```python
from build123d import *

# Parameters (mm, degrees)
F0_R      = 1.5
F0_R_2    = 11.7126871306
F1_DEPTH  = 4
F2_R      = 4
F3_DEPTH  = 15
F6_DEPTH  = 0.6
F7_W      = 42.3
F7_H      = 22
F8_DEPTH  = 5
F11_R     = 1.0444740365
F12_DEPTH = 5
F14_R     = 1.0444740365
F15_DEPTH = 5
F16_W     = 6.0576063115
F16_H     = 10.3428596631
F16_R     = 1.0444740365
F17_DEPTH = 6
F18_SIZE  = 5.99999
F19_R     = 1.4573614865
F20_DEPTH = 7
F21_W     = 1.9849594682
F21_H     = 5.3345812485
F22_DEPTH = 5
F23_W     = 6.0576063115
F23_H     = 5.2529345267
F24_DEPTH = 1


# Not quite as in the source:
# - a fillet or chamfer is up to 0.001 mm smaller than in the source, because OpenCascade refuses the exact size


with BuildPart() as f1:
    # F0 (on Top) → F1 (new body)
    with BuildSketch(Plane.XY):
        with BuildLine():
            Line((21.15, -21.15), (21.15, 21.15))
            Line((21.15, 21.15), (8.5471369535, 21.15))
            ThreePointArc((8.5471369535, 21.15), (6.0437384995, 27.1937384995), (0, 29.6971369535))
            ThreePointArc((0, 29.6971369535), (-6.0437384995, 27.1937384995), (-8.5471369535, 21.15))
            Line((-8.5471369535, 21.15), (-21.15, 21.15))
            Line((-21.15, 21.15), (-21.15, -21.15))
            Line((-21.15, -21.15), (-8.5471369535, -21.15))
            ThreePointArc((-8.5471369535, -21.15), (0, -29.6971369535), (8.5471369535, -21.15))
            Line((8.5471369535, -21.15), (21.15, -21.15))
        make_face()
        with Locations((-15.5, -15.5)):
            Circle(F0_R, mode=Mode.SUBTRACT)
        with Locations((15.5, -15.5)):
            Circle(F0_R, mode=Mode.SUBTRACT)
        with Locations((-15.5, 15.5)):
            Circle(F0_R, mode=Mode.SUBTRACT)
        Circle(F0_R_2, mode=Mode.SUBTRACT)
        with Locations((15.5, 15.5)):
            Circle(F0_R, mode=Mode.SUBTRACT)
    extrude(amount=F1_DEPTH)

    # F2 (on face) → F3 (join)
    with BuildSketch(Plane(origin=(0, 0, 0), x_dir=(1, 0, 0), z_dir=(0, 0, -1))):
        with BuildLine():
            ThreePointArc((-8.5471369535, 21.15), (0, 12.6028630465), (8.5471369535, 21.15))
            ThreePointArc((8.5471369535, 21.15), (0, 29.6971369535), (-8.5471369535, 21.15))
        make_face()
        with Locations((0, 21.15)):
            Circle(F2_R, mode=Mode.SUBTRACT)
        with BuildLine():
            ThreePointArc((-8.5471369535, -21.15), (0, -29.6971369535), (8.5471369535, -21.15))
            ThreePointArc((8.5471369535, -21.15), (0, -12.6028630465), (-8.5471369535, -21.15))
        make_face()
        with Locations((0, -21.15)):
            Circle(F2_R, mode=Mode.SUBTRACT)
    extrude(amount=F3_DEPTH)

    # F7 (on face) → F8 (join)
    with BuildSketch(Plane(origin=(-21.15, 0, 0), x_dir=(0, -1, 0), z_dir=(-1, 0, 0))):
        with Locations((0, 11)):
            Rectangle(F7_W, F7_H)
    extrude(amount=F8_DEPTH)

    # F9: union 


with BuildPart() as f6:
    # F5 (on offset) → F6 (new body)
    with BuildSketch(Plane(origin=(-21.15, 0, 0), x_dir=(0, -1, 0), z_dir=(-1, 0, 0))):
        Polygon((-10, 17.4662213922), (-20, -0.5337786078), (10, -0.5337786078), (20, 17.4662213922), align=None)
    extrude(amount=F6_DEPTH)


with BuildPart() as f1_1:
    add(f1.part)

    # F10: cut F6
    add(f6.part, mode=Mode.SUBTRACT)

    # F11 (on face) → F12 (join)
    with BuildSketch(Plane.YZ.offset(21.15)):
        with BuildLine():
            Line((-4.4944686815, -1.2040658621), (-4.4944686815, 0))
            Line((-4.4944686815, 0), (-8.6928773671, 0))
            Line((-8.6928773671, 0), (-8.6928773671, -1.2551693944))
            ThreePointArc((-8.6928773671, -1.2551693944), (-6.5681212582, -3.3288219711), (-4.4944686815, -1.2040658621))
        make_face()
        with Locations((-6.5936730243, -1.4166244073)):
            Circle(F11_R, mode=Mode.SUBTRACT)
    extrude(amount=-F12_DEPTH)

    # F14 (on offset) → F15 (join)
    with BuildSketch(Plane(origin=(-17.25, 0, 0), x_dir=(0, -1, 0), z_dir=(-1, 0, 0))):
        with BuildLine():
            Line((8.6928773671, -1.2551693944), (8.6928773671, 0))
            Line((8.6928773671, 0), (4.4944686815, 0))
            Line((4.4944686815, 0), (4.4944686815, -1.2040658621))
            ThreePointArc((4.4944686815, -1.2040658621), (6.5681212582, -3.3288219711), (8.6928773671, -1.2551693944))
        make_face()
        with Locations((6.5936730243, -1.4166244073)):
            Circle(F14_R, mode=Mode.SUBTRACT)
    extrude(amount=-F15_DEPTH)

    # F16 (on face) → F17 (join)
    with BuildSketch(Plane(origin=(-26.15, 0, 0), x_dir=(0, -1, 0), z_dir=(-1, 0, 0))):
        with Locations((6.7643582588, 0.7691108622)):
            Rectangle(F16_W, F16_H)
        with BuildLine():
            ThreePointArc((8.6928773671, -1.2551693944), (6.5681212582, -3.3288219711), (4.4944686815, -1.2040658621))
            Line((4.4944686815, -1.2040658621), (4.4944686815, 0))
            Line((4.4944686815, 0), (8.6928773671, 0))
            Line((8.6928773671, 0), (8.6928773671, -1.2551693944))
        make_face(mode=Mode.SUBTRACT)
        with BuildLine():
            ThreePointArc((8.6928773671, -1.2551693944), (6.5681212582, -3.3288219711), (4.4944686815, -1.2040658621))
            Line((4.4944686815, -1.2040658621), (4.4944686815, 0))
            Line((4.4944686815, 0), (3.735555103, 0))
            Line((3.735555103, 0), (3.735555103, -4.4023189694))
            Line((3.735555103, -4.4023189694), (9.7931614146, -4.4023189694))
            Line((9.7931614146, -4.4023189694), (9.7931614146, 0))
            Line((9.7931614146, 0), (8.6928773671, 0))
            Line((8.6928773671, 0), (8.6928773671, -1.2551693944))
        make_face()
        with BuildLine():
            Line((4.4944686815, 0), (4.4944686815, -1.2040658621))
            ThreePointArc((4.4944686815, -1.2040658621), (6.5681212582, -3.3288219711), (8.6928773671, -1.2551693944))
            Line((8.6928773671, -1.2551693944), (8.6928773671, 0))
            Line((8.6928773671, 0), (4.4944686815, 0))
        make_face()
        with Locations((6.5936730243, -1.4166244073)):
            Circle(F16_R, mode=Mode.SUBTRACT)
    extrude(amount=F17_DEPTH)

    # F18 (size 6 in the source; OpenCascade refuses exactly that, so slightly less here)
    f18_edges = [f1_1.edges().sort_by_distance(p)[0] for p in [
        (-32.15, -6.764358, 5.940541),
    ]]
    chamfer(f18_edges, length=F18_SIZE)

    # F19 (on face) → F20 (cut)
    with BuildSketch(Plane(origin=(-32.15, 0, 0), x_dir=(0, -1, 0), z_dir=(-1, 0, 0))):
        with Locations((6.5936730243, -1.4166244073)):
            Circle(F19_R)
    extrude(amount=-F20_DEPTH, mode=Mode.SUBTRACT)

    # F21 (on face) → F22 (cut)
    with BuildSketch(Plane(origin=(0, 0, -4.4023189694), x_dir=(1, 0, 0), z_dir=(0, 0, -1))):
        with Locations((-29.0259411559, 6.7643583752)):
            Rectangle(F21_W, F21_H)
    extrude(amount=-F22_DEPTH, mode=Mode.SUBTRACT)

    # F23 (on face) → F24 (cut)
    with BuildSketch(Plane.YZ.offset(-26.15)):
        with Locations((-6.7643582588, -2.6264672633)):
            Rectangle(F23_W, F23_H)
    extrude(amount=-F24_DEPTH, mode=Mode.SUBTRACT)


solid = f1_1.part
```
The listing builds one solid part. Answer for the finished solid, in the listing's coordinates (mm). A direction names the side the tool comes from. Give positions to 0.01 mm unless a question says otherwise; leave off trailing zeros. Order: outer loops, then holes, each group sorted by start corner. A loop starts at its lowest first (then second) coordinate and runs counter-clockwise, first axis right, second up. Notation, with made-up numbers: (38, 67.25) -> (45, 67.25) arc R19 cw to (45, 99.25) -> close; hole circle Ø7 at (89, 31.5). An arc over 180 degrees is marked (long way). Answer as CSV lines item,"result". Start each with the question number.
Q1. A cutting plane is placed at C-C (x = -5). Determine the outline of the cut face in (y, z), then the cut area to 3 significant figures.
Q2. Determine the mould class of faces 6 (the cylindrical face through (-14.785, -7.559, -1.817)), 7 (the flat face through (15, 21.15, 2)), 8 (the flat face through (-24, 0, 22)) for opening direction Y: pulls with the +Y half, pulls with the -Y half, needs draft (parallel to the pull), parting line crosses it, or undercut.
Q3. Which of the six approach directions +Z, -Z, +X, -X, +Y, -Y give full straight-line access (tool end or side, diameter ignored) to faces 1 (the cylindrical face through (-31.099, -5.138, -1.353)), 2 (the cylindrical face through (3.8, -22.4, -7.4)), 3 (the flat face through (16.15, -8, -2)), 4 (the flat face through (15, -21.15, 2)), 5 (the flat face through (-23, 21.15, 6))?
Q4. A cutting plane is placed at A-A (x = -15.5). Determine the outline of the cut face in (y, z), then the cut area to 3 significant figures.
Q5. Given pin 1 (4 mm diameter, centred on x = -1.5, y = 21, fed in from -Z); pin 2 (1.3 mm diameter, centred on y = -6.5, z = -1.5, fed in from +X); pin 3 (12 mm diameter, centred on x = -0.5, y = 14.5, fed in from +Z); pin 4 (2 mm diameter, centred on x = -29, z = -3, fed in from -Y), each flat-ended and moving along its own axis, determine where each tip first touches the part or whether it passes through.
Q6. Find the intervals of material crossed by L1, parallel to Y at x = 0, z = -4.5; L2, parallel to X at y = 21, z = -5; L3, parallel to Y at x = -15.5, z = 1.3, in increasing order.
Q7. A cutting plane is placed at D-D (z = 13.5). Determine the outline of the cut face in (x, y), then the cut area to 4 significant figures.
Q8. A cutting plane is placed at B-B (y = 0). Determine the outline of the cut face in (x, z).
Results found:
1,outline,"(-28.08, -15) -> (-14.22, -15) -> (-14.22, 0) -> (-10.59, 0) -> (-10.59, 4) -> (-28.08, 4) -> close; (10.59, 0) -> (14.22, 0) -> (14.22, -15) -> (28.08, -15) -> (28.08, 4) -> (10.59, 4) -> close"
1,area,"556 mm2"
2,face 6,"undercut"
2,face 7,"pulls with the +Y half"
2,face 8,"needs draft"
3,face 1,"-X"
3,face 2,"-Z"
3,face 3,"-Z, +Y, -Y"
3,face 4,"+Z, -Z, +X, -Y"
3,face 5,"+Z, -Z, -X, +Y"
4,outline,"(-21.15, 0) -> (-17, 0) -> (-17, 4) -> (-21.15, 4) -> close; (-14, 0) -> (-8.69, 0) -> (-8.69, -1.26) arc R2.1 ccw to (-4.49, -1.2) -> (-4.49, 0) -> (14, 0) -> (14, 4) -> (-14, 4) -> close; (17, 0) -> (21.15, 0) -> (21.15, 4) -> (17, 4) -> close; hole circle Ø2.09 at (-6.59, -1.42)"
4,area,"154 mm2"
5,pin 1,"z = 0"
5,pin 2,"through"
5,pin 3,"z = 4"
5,pin 4,"y = -9.79"
6,L1,"-29.7 to -25.15, -17.15 to -12.6, 12.6 to 17.15, 25.15 to 29.7"
6,L2,"-8.55 to -4, 4 to 8.55"
6,L3,"-21.15 to -17, -14 to 14, 17 to 21.15"
7,outline,"(-26.15, -21.15) -> (-21.15, -21.15) -> (-21.15, -17.8) -> (-21.75, -17.8) -> (-21.75, 12.2) -> (-21.15, 12.2) -> (-21.15, 21.15) -> (-26.15, 21.15) -> close"
7,area,"193.5 mm2"
8,outline,"(-26.15, 0) -> (-21.75, 0) -> (-21.75, 17.47) -> (-21.15, 17.47) -> (-21.15, 22) -> (-26.15, 22) -> close; (-21.15, 0) -> (-11.71, 0) -> (-11.71, 4) -> (-21.15, 4) -> close; (11.71, 0) -> (21.15, 0) -> (21.15, 4) -> (11.71, 4) -> close"
